Verification items for the finished model (mm, model axes). Face numbers are marked on the shaded views. A direction names the side the tool comes from. Coordinates: 2 decimals unless noted, no trailing zeros. Write each loop counter-clockwise with the first axis right and the second up, starting at its lowest first coordinate (ties: lowest second). Pieces come first, ordered by that corner, then holes. Notation, with made-up numbers: (84, 44.5) -> (117, 44.5) arc R16 ccw to (117, 52.5) -> close; hole circle Ø5 at (78.5, 65.25). An arc over 180 degrees is marked (long way). Use CSV: the item, a comma, the result in double quotes.
```python
from build123d import *

# Parameters (mm, degrees)
SKETCH1_R           = 6.125
SKETCH1_W           = 2.5
SKETCH1_H           = 2.5
BOSS_EXTRUDE1_DEPTH = 1.5
SKETCH1_2_W         = 2.5
SKETCH1_2_H         = 2.5
BOSS_EXTRUDE2_DEPTH = 26


with BuildPart() as part:
    # Sketch1 → Boss-Extrude1 (new body)
    with BuildSketch(Plane(origin=(0, 0, 0), x_dir=(1, 0, 0), z_dir=(0, 1, 0))):
        with Locations(Location((0, 0, 0), (0, 0, 270))):
            Circle(SKETCH1_R)
        Rectangle(SKETCH1_W, SKETCH1_H, mode=Mode.SUBTRACT)
    extrude(amount=BOSS_EXTRUDE1_DEPTH)

    # Sketch1_2 → Boss-Extrude2 (add)
    with BuildSketch(Plane(origin=(0, 0, 0), x_dir=(1, 0, 0), z_dir=(0, 1, 0))):
        Rectangle(SKETCH1_2_W, SKETCH1_2_H)
    extrude(amount=BOSS_EXTRUDE2_DEPTH)


solid = part.part
```
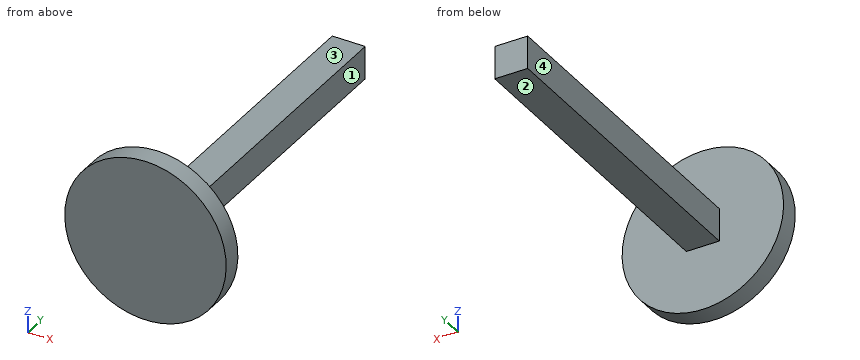
1) Cross-section at B-B (z = 0). Record the boundary of the cut face in (x, y) (3 decimals), plus the area to 3 significant figures.
Return value:
outline,"(-6.125, 0) -> (6.125, 0) -> (6.125, 1.5) -> (1.25, 1.5) -> (1.25, 26) -> (-1.25, 26) -> (-1.25, 1.5) -> (-6.125, 1.5) -> close"
area,"79.6 mm2"
2) Scan lines: L1, parallel to X at y = 3.75, z = 0.5; L2, parallel to Y at x = 2, z = -0.75. Record each from-to range of solid material in increasing order.
Return value:
L1,"-1.25 to 1.25"
L2,"0 to 1.5"
3) Cross-section at A-A (x = 0). Record the boundary of the cut face in (y, z) (3 decimals).
Return value:
outline,"(0, -6.125) -> (1.5, -6.125) -> (1.5, -1.25) -> (26, -1.25) -> (26, 1.25) -> (1.5, 1.25) -> (1.5, 6.125) -> (0, 6.125) -> close"
4) Gauge pin test, flat ends, axial feed: pin 1 (1.5 mm diameter, centred on y = 12.5, z = -2.5, fed in from -X); pin 2 (4 mm diameter, centred on x = 0.5, z = 2, fed in from +Y); pin 3 (4 mm diameter, centred on x = -4, z = -2.5, fed in from +Y); pin 4 (3 mm diameter, centred on x = -0.5, y = 8, fed in from +Z). Record the tip position at first contact, or that the pin passes through.
Return value:
pin 1,"through"
pin 2,"y = 26"
pin 3,"y = 1.5"
pin 4,"z = 1.25"
5) Cross-section at D-D (x = 3). Record the boundary of the cut face in (y, z), plus the area to 3 significant figures.
Return value:
outline,"(0, -5.34) -> (1.5, -5.34) -> (1.5, 5.34) -> (0, 5.34) -> close"
area,"16.0 mm2"
6) Set-up check for the marked faces 1, 2, 3 and 4: record each of +Z, -Z, +X, -X, +Y, -Y from which the full face is reachable in a straight line by a thin tool's end or side.
Return value:
face 1,"+Z, -Z, +X, +Y"
face 2,"-Z, +X, -X, +Y"
face 3,"+Z, +X, -X, +Y"
face 4,"+Z, -Z, -X, +Y"
7) Cross-section at C-C (y = 18). Record the boundary of the cut face in (x, z).
Return value:
outline,"(-1.25, -1.25) -> (1.25, -1.25) -> (1.25, 1.25) -> (-1.25, 1.25) -> close"
